Read the model definition and answer for the solid it produces. Units are mm, in the model's axes. A direction names the side the tool comes from. Round coordinates to 2 decimals unless told otherwise and drop trailing zeros. Write each loop counter-clockwise with the first axis right and the second up, starting at its lowest first coordinate (ties: lowest second). Pieces come first, ordered by that corner, then holes. Notation, with made-up numbers: (80.25, 14) - (86.25, 14) arc R12 ccw to (86.25, 28) - close; hole circle Ø11 at (70, -26.75). An arc over 180 degrees is marked (long way). Use one line per item in the form item = value. Start each with the question number.
1) The part is cut by section D-D, the plane x = -5. Give the vertices of the cut face in (y, z).
2) The part is cut by section A-A, the plane z = -8.75. Give the vertices of the cut face in (x, y), plus the area to 3 significant figures.
3) For a pull along X with two mould halves and no side action, classify faces 1 (the face through (9.5, -1, -7)), 2 (the face through (-12.5, -1, -5)), 3 (the face through (12.5, -1, -5)) as released by +X, released by -X, zero draft, split by the parting line, or undercut.
4) The part is cut by section B-B, the plane y = -1.4. Give the vertices of the cut face in (x, z), plus the area to 3 significant figures.
5) This flat-tipped pin is pushed along its axis until it touches: pin 1 (3 mm diameter, centred on x = -1.5, z = -4, fed in from -Y). Where does it stop, or does it pass through?
6) Consider line 1 along X through (y, z) = (-2.3, -8.75); line 2 along X through (y, z) = (-1, -4.5); line 3 along Z through (x, y) = (-6, -0.8). Determine where each line is inside the solid, lowest interval first. Write a range as from..to.
7) The part is cut by section C-C, the plane z = -4.25. Give the vertices of the cut face in (x, y).
8) For faces 4 (the face through (8.9, -1.52, -3.57)), 5 (the face through (0.2, -3, -2.8)), determine the directions among +Z, -Z, +X, -X, +Y, -Y from which every point of the face is accessible in a straight line to the end or side of a thin tool.
from build123d import *

# Parameters (mm, degrees)
SALIENTE_EXTRUIR1_DEPTH = 3
REDONDEO4_R             = 2
REDONDEO5_R             = 2


with BuildPart() as part:
    # Croquis1 → Saliente-Extruir1 (new body)
    with BuildSketch(Plane(origin=(0, 0, 0), x_dir=(1, 0, 0), z_dir=(0, 1, 0))):
        Polygon((12.5, 0), (-12.5, 0), (-12.5, 10), (-9.5, 10), (-9.5, 3), (9.5, 3), (9.5, 10), (12.5, 10), align=None)
    extrude(amount=-SALIENTE_EXTRUIR1_DEPTH)

    # Redondeo4
    redondeo4_edges = [part.edges().sort_by_distance(p)[0] for p in [
        (-9.5, -1.5, -3),
    ]]
    fillet(redondeo4_edges, radius=REDONDEO4_R)

    # Redondeo5
    redondeo5_edges = [part.edges().sort_by_distance(p)[0] for p in [
        (9.5, -1.5, -3),
    ]]
    fillet(redondeo5_edges, radius=REDONDEO5_R)


solid = part.part
Geometry results:
q1.outline = (-3, -3) - (0, -3) - (0, 0) - (-3, 0) - close
q2.outline = (-12.5, -3) - (-9.5, -3) - (-9.5, 0) - (-12.5, 0) - close; (9.5, -3) - (12.5, -3) - (12.5, 0) - (9.5, 0) - close
q2.area = 18.0 mm2
q3.face_1 = undercut
q3.face_2 = released by -X
q3.face_3 = released by +X
q4.outline = (-12.5, -10) - (-9.5, -10) - (-9.5, -5) arc R2 cw to (-7.5, -3) - (7.5, -3) arc R2 cw to (9.5, -5) - (9.5, -10) - (12.5, -10) - (12.5, 0) - (-12.5, 0) - close
q4.area = 119 mm2
q5.pin_1 = -3
q6.line_1 = -12.5..-9.5, 9.5..12.5
q6.line_2 = -12.5..-9.44, 9.44..12.5
q6.line_3 = -3..0
q7.outline = (-12.5, -3) - (-9.35, -3) - (-9.35, 0) - (-12.5, 0) - close; (9.35, -3) - (12.5, -3) - (12.5, 0) - (9.35, 0) - close
q8.face_4 = -Z, +Y, -Y
q8.face_5 = +Z, -Z, +X, -X, -Y
